Part print with two shaded views. Sizes in mm from the minimum x, y, z corner. Round coordinates to 2 decimals unless told otherwise and drop trailing zeros. Write each loop counter-clockwise with the first axis right and the second up, starting at its lowest first coordinate (ties: lowest second). Pieces come first, ordered by that corner, then holes.
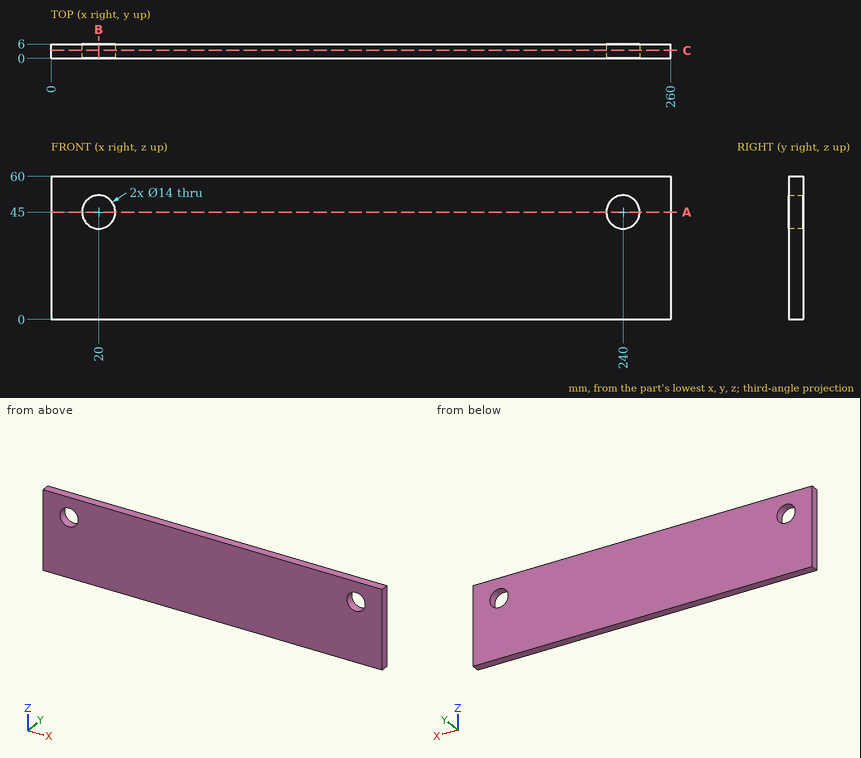
Q1. Cut at B-B on x = 20. Write the cut outline in (y, z).
Values follow:
outline: (0, 0) - (6, 0) - (6, 38) - (0, 38) - close; (0, 52) - (6, 52) - (6, 60) - (0, 60) - close
Q2. Cut at C-C on y = 3.35. Write the cut outline in (x, z), plus the area to 3 significant figures.
Values follow:
outline: (0, 0) - (260, 0) - (260, 60) - (0, 60) - close; hole circle Ø14 at (20, 45); hole circle Ø14 at (240, 45)
area: 15,300 mm2
Q3. Cut at A-A on z = 45. Write the cut outline in (x, y), plus the area to 3 significant figures.
Values follow:
outline: (0, 0) - (13, 0) - (13, 6) - (0, 6) - close; (27, 0) - (233, 0) - (233, 6) - (27, 6) - close; (247, 0) - (260, 0) - (260, 6) - (247, 6) - close
area: 1,390 mm2
Q4. Wall check: L1, parallel to X at y = 1.7, z = 45. Give the ranges that are in metal, low to high.
Values follow:
L1: x = 0 to 13, 27 to 233, 247 to 260
